Part model, mm, in its own coordinate system. A direction names the side the tool comes from. Round coordinates to 2 decimals unless told otherwise and drop trailing zeros. Write each loop counter-clockwise with the first axis right and the second up, starting at its lowest first coordinate (ties: lowest second). Pieces come first, ordered by that corner, then holes. Notation, with made-up numbers: M -29.75,-3 L 16.25,-3 A37 cw 16.25,33 Z; hole C 69.25,-28 d9. An arc over 180 degrees is marked long. Use one line per item in the form item = value. Start each with the question number.
Item 1: Mould opens along Z. For faces 4 (the face through (-9.02, -3.54, 0.39)), 5 (the face through (-6.064, -6.096, 3.631)), 6 (the face through (-6.06, -6.2, -4.68)), 7 (the face through (-13.952, -6, -1)) say: +Z half, -Z half, draft (parallel to the pull), parting line (faces both ways), or undercut.
Item 2: Cut at C-C, the plane x = -0.25. Give the cut face in (y, z), then the cut area to 3 significant figures.
Item 3: Which spindle directions (+Z, -Z, +X, -X, +Y, -Y) get a long thin tool onto all of the face, cutting with end or side? Do faces 1 (the face through (-1.167, -4.93, 1.636)), 2 (the face through (-3.952, -2, 0)), 3 (the face through (-6, -10, 0)). Say none if no direction does.
Item 4: Cut at B-B, the plane y = -2.5. Give the cut face in (x, z), then the cut area to 3 significant figures.
Item 5: Flat gauge pins, fed straight in: pin 1 Ø4 at (x, z) = (-0.95, 0) entering from -Y; pin 2 Ø4 at (x, z) = (-7, -4.5) entering from -Y; pin 3 Ø6 at (x, y) = (-6, -8.5) entering from +Z; pin 4 Ø5 at (x, y) = (-9, -3.5) entering from +Z. Where does each tip first touch, or does it go through?
Item 6: Cut at D-D, the plane z = -5.25. Give the cut face in (x, y).
Item 7: Probe L1, parallel to Z at x = -5.75, y = -2.3; L2, parallel to Z at x = 0.25, y = -10.75; L3, parallel to Z at x = -1.75, y = -1.75. List the from-to ranges inside material, lowest first.
Item 8: Cut at A-A, the plane x = -9.25. Give the cut face in (y, z), then the cut area to 3 significant figures.
from build123d import *

# Parameters (mm, degrees)
F0_W     = 16
F0_H     = 12
F0_R     = 1.65
F1_DEPTH = 13
F2_W     = 16
F2_H     = 10
F2_R     = 1.65
F3_DEPTH = 3
F5_DEPTH = 16.001
F6_R     = 1.3
F7_DEPTH = 10


with BuildPart() as f1:
    # F0 (on Front) → F1 (new body)
    with BuildSketch(Plane.XZ):
        with Locations((-5.952034, -1)):
            Rectangle(F0_W, F0_H)
        with Locations((-0.952034, 0)):
            Circle(F0_R, mode=Mode.SUBTRACT)
    extrude(amount=F1_DEPTH)

    # F2 (on face) → F3 (cut)
    with BuildSketch(Plane.XZ.offset(13)):
        with Locations((-5.952034, 0)):
            Rectangle(F2_W, F2_H)
        with Locations((-0.952034, 0)):
            Circle(F2_R, mode=Mode.SUBTRACT)
    extrude(amount=-F3_DEPTH, mode=Mode.SUBTRACT)

    # F4 (on face) → F5 (cut, through all)
    with BuildSketch(Plane(origin=(-13.952034, 0, 0), x_dir=(0, -1, 0), z_dir=(-1, 0, 0))):
        with BuildLine():
            ThreePointArc((0, 0), (0.673654, 1.626346), (2.3, 2.3))
            Line((2.3, 2.3), (10, 5))
            Line((10, 5), (0, 5))
            Line((0, 5), (0, 0))
        make_face()
        with BuildLine():
            Line((10, -7), (2.3, -2.3))
            ThreePointArc((2.3, -2.3), (0.673654, -1.626346), (0, 0))
            Line((0, 0), (0, -7))
            Line((0, -7), (10, -7))
        make_face()
    extrude(amount=-F5_DEPTH, mode=Mode.SUBTRACT)

    # F6 (on face) → F7 (cut)
    with BuildSketch(Plane(origin=(-13.952034, 0, 0), x_dir=(0, -1, 0), z_dir=(-1, 0, 0))):
        with Locations((2.3, 0)):
            Circle(F6_R)
    extrude(amount=-F7_DEPTH, mode=Mode.SUBTRACT)


solid = f1.part
Model answer:
q1.face_4 = undercut
q1.face_5 = +Z half
q1.face_6 = -Z half
q1.face_7 = draft
q2.outline = M -13,-7 L -10,-7 L -2.3,-2.3 A2.3 ccw -0.55,-1.49 L -10,-1.49 L -10,-5 L -13,-5 Z; M -10,1.49 L -0.55,1.49 A2.3 ccw -2.3,2.3 L -10,5 Z
q2.area = 48.9 mm²
q3.face_1 = +Y, -Y
q3.face_2 = -X
q3.face_3 = +Z, +X, -X, -Y
q4.outline = M -13.95,-2.42 L 2.05,-2.42 L 2.05,2.37 L -13.95,2.37 L -13.95,1.28 L -3.95,1.28 L -3.95,-1.28 L -13.95,-1.28 Z; hole C -0.95,0 d3.3
q4.area = 42.4 mm²
q5.pin_1 = -10
q5.pin_2 = -13
q5.pin_3 = 5
q5.pin_4 = 3.6
q6.outline = M -13.95,-13 L 2.05,-13 L 2.05,-7.13 L -13.95,-7.13 Z
q7.L1 = -2.3 to -1.3, 1.3 to 2.3
q7.L2 = -7 to -5
q7.L3 = -2.23 to -1.44, 1.44 to 2.23
q8.outline = M -13,-7 L -10,-7 L -2.3,-2.3 A2.3 ccw 0,0 A2.3 ccw -2.3,2.3 L -10,5 L -10,-5 L -13,-5 Z; hole C -2.3,0 d2.6
q8.area = 72.9 mm²
